from build123d import *

# Parameters (mm, degrees)
ESQUISSE1_W              = 52
ESQUISSE1_H              = 30
BOSS_EXTRU_1_DEPTH       = 2
EMPREINTE2_OUTLINE_W     = 2
EMPREINTE2_OUTLINE_H     = 2
EMPREINTE2_OUTLINE_W_2   = 2.02
EMPREINTE2_DEPTH         = 7.575
EMPREINTE2_START         = 22.725
EMPREINTE2_2_OUTLINE_W   = 2
EMPREINTE2_2_OUTLINE_H   = 2
EMPREINTE2_2_OUTLINE_W_2 = 2.02
EMPREINTE2_2_DEPTH       = 7.275


# Read off the part's stored shape, not the designer's step: Empreinte2
with BuildPart() as part:
    # Esquisse1 → Boss.-Extru.1 (new body)
    with BuildSketch(Plane.XY):
        with Locations((26, 15)):
            Rectangle(ESQUISSE1_W, ESQUISSE1_H)
    extrude(amount=BOSS_EXTRU_1_DEPTH)

    # Empreinte2 outline → Empreinte2 (cut)
    with BuildSketch(Plane(origin=(0, 0, 0), x_dir=(1, 0, 0), z_dir=(0, 1, 0))):
        with Locations((51, -1)):
            Rectangle(EMPREINTE2_OUTLINE_W, EMPREINTE2_OUTLINE_H)
        with Locations((1.01, -1)):
            Rectangle(EMPREINTE2_OUTLINE_W_2, EMPREINTE2_OUTLINE_H)
    extrude(amount=EMPREINTE2_DEPTH, mode=Mode.SUBTRACT)

    # Empreinte2 2 outline → Empreinte2 2 (cut)
    with BuildSketch(Plane(origin=(0, 0, 0), x_dir=(1, 0, 0), z_dir=(0, 1, 0)).offset(EMPREINTE2_START)):
        with Locations((51, -1)):
            Rectangle(EMPREINTE2_2_OUTLINE_W, EMPREINTE2_2_OUTLINE_H)
        with Locations((1.01, -1)):
            Rectangle(EMPREINTE2_2_OUTLINE_W_2, EMPREINTE2_2_OUTLINE_H)
    extrude(amount=EMPREINTE2_2_DEPTH, mode=Mode.SUBTRACT)


solid = part.part
Can you work these out from the model? Positions are in its coordinate system, mm. A direction names the side the tool comes from. Round coordinates to 2 decimals unless told otherwise and drop trailing zeros. Loops run counter-clockwise (first coordinate to the right, second up) from the corner with the lowest first, then second, coordinate; pieces in that order, holes last. Notation, with made-up numbers: (1.25, -24.75) - (8.25, -24.75) arc R19 cw to (8.25, -15.75) - close; hole circle Ø4 at (15.5, 25.25). An arc over 180 degrees is marked (long way). Write item = value, one per line. Start each with the question number.
(1) For P1, Ø1, axis at y = 26, z = 1, coming from the -X side; P2, Ø1, axis at y = 25, z = 1.5, coming from the +X side; P3, Ø0.6, axis at x = 51, z = 0.5, coming from the -Y side (3 decimals), each with a flat end and sliding along its axis, tell me the tip position at first contact or that it passes through.
(2) If I drill on probe 1 along X at (y, z) = (26.75, 0.6), over which ranges is the centre line in solid material (lowest first)? Write a range as [from, to].
(3) For faces 1 (the face through (2.02, 26, 1)), 2 (the face through (1, 7.575, 1)), 3 (the face through (50, 26, 1)), 4 (the face through (52, 15, 1)), 5 (the face through (50, 4, 1)), which set-ups out of +Z, -Z, +X, -X, +Y, -Y let a thin tool reach every point of the face, with its end or its side?
(4) If we section it at A-A (z = 1.3): Please give me the cut outline in (x, y) (3 decimals).
(5) If we section it at B-B (y = 4.5): Please give me the cut outline in (x, z).
Ans:
q1.P1 = 2.02
q1.P2 = 50
q1.P3 = 7.575
q2.probe_1 = [2.02, 50]
q3.face_1 = +Z, -Z, -X, +Y
q3.face_2 = +Z, -Z, -X, -Y
q3.face_3 = +Z, -Z, +X, +Y
q3.face_4 = +Z, -Z, +X, +Y, -Y
q3.face_5 = +Z, -Z, +X, -Y
q4.outline = (0, 7.575) - (2.02, 7.575) - (2.02, 0) - (50, 0) - (50, 7.575) - (52, 7.575) - (52, 22.725) - (50, 22.725) - (50, 30) - (2.02, 30) - (2.02, 22.725) - (0, 22.725) - close
q5.outline = (2.02, 0) - (50, 0) - (50, 2) - (2.02, 2) - close
